from build123d import *

# Parameters (mm, degrees)
SKETCH_1_W          = 40
SKETCH_1_H          = 15
SKETCH_1_W_2        = 38
SKETCH_1_H_2        = 13
EXTRUDE_1_DEPTH     = 1100
SKETCH_2_R          = 3.575
SKETCH_2_R_2        = 1.6
CUT_EXTRUDE_1_DEPTH = 1101.829232897
SKETCH_3_R          = 1.575
CUT_EXTRUDE_2_DEPTH = 1101.829232897
SKETCH_6_R          = 13
CUT_EXTRUDE_4_DEPTH = 1101.829232897
SKETCH_7_R          = 1.6
CUT_EXTRUDE_5_DEPTH = 1101.829232897


with BuildPart() as part:
    # Sketch 1 → Extrude 1 (new body)
    with BuildSketch(Plane.XY):
        with Locations((20, 7.5)):
            Rectangle(SKETCH_1_W, SKETCH_1_H)
        with Locations((20, 7.5)):
            Rectangle(SKETCH_1_W_2, SKETCH_1_H_2, mode=Mode.SUBTRACT)
    extrude(amount=EXTRUDE_1_DEPTH)

    # Sketch 2 → Cut-Extrude 1 (cut, through all)
    with BuildSketch(Plane(origin=(0, 15, 0), x_dir=(1, 0, 0), z_dir=(0, 1, 0))):
        with Locations(Location((12, -21, 0), (0, 0, 270))):
            Circle(SKETCH_2_R)
        with Locations(Location((28, -21, 0), (0, 0, 270))):
            Circle(SKETCH_2_R)
        with Locations(Location((33, -498, 0), (0, 0, 270))):
            Circle(SKETCH_2_R_2)
        with Locations(Location((7, -522, 0), (0, 0, 270))):
            Circle(SKETCH_2_R_2)
        with Locations(Location((33, -522, 0), (0, 0, 270))):
            Circle(SKETCH_2_R_2)
        with Locations(Location((7, -590, 0), (0, 0, 270))):
            Circle(SKETCH_2_R_2)
        with Locations(Location((7, -510, 0), (0, 0, 270))):
            Circle(SKETCH_2_R_2)
        with Locations(Location((33, -590, 0), (0, 0, 270))):
            Circle(SKETCH_2_R_2)
        with Locations(Location((33, -510, 0), (0, 0, 270))):
            Circle(SKETCH_2_R_2)
        with Locations(Location((7, -602, 0), (0, 0, 270))):
            Circle(SKETCH_2_R_2)
        with Locations(Location((33, -602, 0), (0, 0, 270))):
            Circle(SKETCH_2_R_2)
        with Locations(Location((7, -498, 0), (0, 0, 270))):
            Circle(SKETCH_2_R_2)
        with Locations(Location((7, -578, 0), (0, 0, 270))):
            Circle(SKETCH_2_R_2)
        with Locations(Location((33, -578, 0), (0, 0, 270))):
            Circle(SKETCH_2_R_2)
        with Locations(Location((12, -77, 0), (0, 0, 270))):
            Circle(SKETCH_2_R)
        with Locations(Location((28, -77, 0), (0, 0, 270))):
            Circle(SKETCH_2_R)
        with Locations(Location((12, -1023, 0), (0, 0, 270))):
            Circle(SKETCH_2_R)
        with Locations(Location((28, -1023, 0), (0, 0, 270))):
            Circle(SKETCH_2_R)
        with Locations(Location((28, -1079, 0), (0, 0, 270))):
            Circle(SKETCH_2_R)
        with Locations(Location((12, -1079, 0), (0, 0, 270))):
            Circle(SKETCH_2_R)
    extrude(amount=-CUT_EXTRUDE_1_DEPTH, mode=Mode.SUBTRACT)

    # Sketch 3 → Cut-Extrude 2 (cut, through all)
    with BuildSketch(Plane(origin=(0, 15, 0), x_dir=(1, 0, 0), z_dir=(0, 1, 0))):
        with Locations(Location((24, -629, 0), (0, 0, 270))):
            Circle(SKETCH_3_R)
        with Locations(Location((36, -629, 0), (0, 0, 270))):
            Circle(SKETCH_3_R)
        with Locations(Location((24, -619, 0), (0, 0, 270))):
            Circle(SKETCH_3_R)
        with Locations(Location((36, -619, 0), (0, 0, 270))):
            Circle(SKETCH_3_R)
        with Locations(Location((36, -641, 0), (0, 0, 270))):
            Circle(SKETCH_3_R)
        with Locations(Location((24, -641, 0), (0, 0, 270))):
            Circle(SKETCH_3_R)
        with Locations(Location((24, -651, 0), (0, 0, 270))):
            Circle(SKETCH_3_R)
        with Locations(Location((36, -651, 0), (0, 0, 270))):
            Circle(SKETCH_3_R)
        with Locations(Location((24, -471, 0), (0, 0, 270))):
            Circle(SKETCH_3_R)
        with Locations(Location((36, -471, 0), (0, 0, 270))):
            Circle(SKETCH_3_R)
        with Locations(Location((24, -481, 0), (0, 0, 270))):
            Circle(SKETCH_3_R)
        with Locations(Location((36, -481, 0), (0, 0, 270))):
            Circle(SKETCH_3_R)
        with Locations(Location((36, -459, 0), (0, 0, 270))):
            Circle(SKETCH_3_R)
        with Locations(Location((24, -459, 0), (0, 0, 270))):
            Circle(SKETCH_3_R)
        with Locations(Location((24, -449, 0), (0, 0, 270))):
            Circle(SKETCH_3_R)
        with Locations(Location((36, -449, 0), (0, 0, 270))):
            Circle(SKETCH_3_R)
    extrude(amount=-CUT_EXTRUDE_2_DEPTH, mode=Mode.SUBTRACT)

    # Sketch 6 → Cut-Extrude 4 (cut, through all)
    with BuildSketch(Plane.XZ):
        with Locations(Location((20, 980, 0), (0, 0, 270))):
            Circle(SKETCH_6_R)
        with Locations(Location((20, 939, 0), (0, 0, 270))):
            Circle(SKETCH_6_R)
        with Locations(Location((20, 898, 0), (0, 0, 270))):
            Circle(SKETCH_6_R)
        with Locations(Location((20, 857, 0), (0, 0, 270))):
            Circle(SKETCH_6_R)
        with Locations(Location((20, 816, 0), (0, 0, 270))):
            Circle(SKETCH_6_R)
        with Locations(Location((20, 775, 0), (0, 0, 270))):
            Circle(SKETCH_6_R)
        with Locations(Location((20, 324, 0), (0, 0, 270))):
            Circle(SKETCH_6_R)
        with Locations(Location((20, 283, 0), (0, 0, 270))):
            Circle(SKETCH_6_R)
        with Locations(Location((20, 242, 0), (0, 0, 270))):
            Circle(SKETCH_6_R)
        with Locations(Location((20, 201, 0), (0, 0, 270))):
            Circle(SKETCH_6_R)
        with Locations(Location((20, 160, 0), (0, 0, 270))):
            Circle(SKETCH_6_R)
        with Locations(Location((20, 119, 0), (0, 0, 270))):
            Circle(SKETCH_6_R)
        with Locations(Location((20, 703, 0), (0, 0, 270))):
            Circle(SKETCH_6_R)
        with Locations(Location((20, 396, 0), (0, 0, 270))):
            Circle(SKETCH_6_R)
    extrude(amount=-CUT_EXTRUDE_4_DEPTH, mode=Mode.SUBTRACT)

    # Sketch 7 → Cut-Extrude 5 (cut, through all)
    with BuildSketch(Plane.ZY):
        with Locations((336, 7)):
            Circle(SKETCH_7_R)
        with Locations((380, 7)):
            Circle(SKETCH_7_R)
        with Locations((388, 7)):
            Circle(SKETCH_7_R)
        with Locations((396, 7)):
            Circle(SKETCH_7_R)
        with Locations((404, 7)):
            Circle(SKETCH_7_R)
        with Locations((359, 7)):
            Circle(SKETCH_7_R)
        with Locations((352, 7)):
            Circle(SKETCH_7_R)
        with Locations((344, 7)):
            Circle(SKETCH_7_R)
        with Locations((696, 7)):
            Circle(SKETCH_7_R)
        with Locations((740, 7)):
            Circle(SKETCH_7_R)
        with Locations((748, 7)):
            Circle(SKETCH_7_R)
        with Locations((756, 7)):
            Circle(SKETCH_7_R)
        with Locations((764, 7)):
            Circle(SKETCH_7_R)
        with Locations((719, 7)):
            Circle(SKETCH_7_R)
        with Locations((712, 7)):
            Circle(SKETCH_7_R)
        with Locations((704, 7)):
            Circle(SKETCH_7_R)
    extrude(amount=-CUT_EXTRUDE_5_DEPTH, mode=Mode.SUBTRACT)


solid = part.part
Part model, mm, in its own coordinate system. A direction names the side the tool comes from. Coordinates: 2 decimals unless noted, no trailing zeros. Loops run counter-clockwise (first coordinate to the right, second up) from the corner with the lowest first, then second, coordinate; pieces in that order, holes last. Notation, with made-up numbers: (40.5, 47) -> (91.5, 47) arc R27 ccw to (91.5, 86) -> close; hole circle Ø8 at (67, 70). An arc over 180 degrees is marked (long way). Use a Markdown table: item, result. Add a question column.
Item 1: Band-saw the part on A-A on z = 283. Write the cut outline in (x, y), plus the area to 3 significant figures.
Item 2: Probe probe 1 along X at (y, z) = (0.5, 1023) (3 decimals); probe 2 along X at (y, z) = (3.75, 526); probe 3 along X at (y, z) = (14.3, 481) (3 decimals). List the from-to ranges inside material, lowest first.
Item 3: Flat gauge pin, fed straight in: P1, Ø21, axis at x = 20, z = 857, coming from the -Y side. Where does the tip first touch, or does it go through?
Item 4: Pull direction X, two halves, no side cores. Call faces 1 (the cylindrical face through (23.9, 0.5, 844.6)), 2 (the cylindrical face through (20.572, 14.493, 295.987)), 3 (the flat face through (20, 15, 542)): +X half, -X half, draft (parallel to the pull), parting line (faces both ways), or undercut.
Item 5: Band-saw the part on B-B on y = 11.25. Write the cut outline in (x, z), plus the area to 3 significant figures.
Item 6: Which spindle directions (+Z, -Z, +X, -X, +Y, -Y) get a long thin tool onto all of the face, cutting with end or side? Do faces 4 (the cylindrical face through (23.9, 14.5, 106.6)), 5 (the flat face through (20, 14, 542)). Say none if no direction does.
Item 7: Band-saw the part on C-C on z = 430. Write the cut outline in (x, y), plus the area to 3 significant figures.
Geometry says:
| question | item | result |
|---|---|---|
| 1 | outline | (0, 0) -> (7, 0) -> (7, 1) -> (1, 1) -> (1, 14) -> (7, 14) -> (7, 15) -> (0, 15) -> close; (33, 0) -> (40, 0) -> (40, 15) -> (33, 15) -> (33, 14) -> (39, 14) -> (39, 1) -> (33, 1) -> close |
| 1 | area | 54.0 mm² |
| 2 | probe 1 | 0 to 8.425, 15.575 to 24.425, 31.575 to 40 |
| 2 | probe 2 | 0 to 1, 39 to 40 |
| 2 | probe 3 | 0 to 22.425, 25.575 to 34.425, 37.575 to 40 |
| 3 | P1 | through |
| 4 | face 1 | undercut |
| 4 | face 2 | undercut |
| 4 | face 3 | draft |
| 5 | outline | (0, 0) -> (1, 0) -> (1, 1100) -> (0, 1100) -> close; (39, 0) -> (40, 0) -> (40, 1100) -> (39, 1100) -> close |
| 5 | area | 2,200 mm² |
| 6 | face 4 | +Y, -Y |
| 6 | face 5 | +Z, -Z |
| 7 | outline | (0, 0) -> (40, 0) -> (40, 15) -> (0, 15) -> close; hole (1, 1) -> (39, 1) -> (39, 14) -> (1, 14) -> close |
| 7 | area | 106 mm² |
